Input: part model. Units: mm. Frame: model coordinates. Face numbers are marked on the shaded views. Round coordinates to 2 decimals unless told otherwise and drop trailing zeros. Write each loop counter-clockwise with the first axis right and the second up, starting at its lowest first coordinate (ties: lowest second). Pieces come first, ordered by that corner, then holes. Notation, with made-up numbers: (4.25, 35) - (24.25, 35) arc R29 ccw to (24.25, 65) - close; hole circle Ø10 at (16, 11). An arc over 180 degrees is marked (long way). One line per item, written item: value. Start each with the question number.
```python
from build123d import *

# Parameters (mm, degrees)
SKETCH1_R           = 100
SKETCH1_R_2         = 72.5
BOSS_EXTRUDE1_DEPTH = 8
SKETCH2_R           = 2.25
CUT_EXTRUDE1_DEPTH  = 8


with BuildPart() as part:
    # Sketch1 → Boss-Extrude1 (new body)
    with BuildSketch(Plane(origin=(0, 0, 0), x_dir=(1, 0, 0), z_dir=(0, 1, 0))):
        Circle(SKETCH1_R)
        Circle(SKETCH1_R_2, mode=Mode.SUBTRACT)
    extrude(amount=BOSS_EXTRUDE1_DEPTH)

    # Sketch2 → Cut-Extrude1 (cut)
    with BuildSketch(Plane(origin=(0, 0, 0), x_dir=(1, 0, 0), z_dir=(0, 1, 0))):
        with Locations((0, 93.125)):
            Circle(SKETCH2_R)
        with Locations((93.125, 0)):
            Circle(SKETCH2_R)
        with Locations((0, -93.125)):
            Circle(SKETCH2_R)
        with Locations((-93.125, 0)):
            Circle(SKETCH2_R)
        with Locations((0, 79.375)):
            Circle(SKETCH2_R)
        with Locations((79.375, 0)):
            Circle(SKETCH2_R)
        with Locations((0, -79.375)):
            Circle(SKETCH2_R)
        with Locations((-79.375, 0)):
            Circle(SKETCH2_R)
    extrude(amount=CUT_EXTRUDE1_DEPTH, mode=Mode.SUBTRACT)


solid = part.part
```
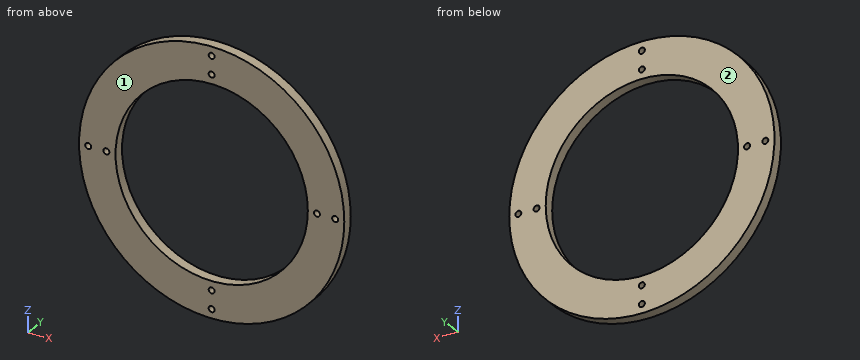
Q1. Cut plane D-D, the plane x = -85. Output: boundary loops of the cut face in (y, z).
Q2. Cut plane B-B, the plane z = 70. Output: boundary loops of the cut face in (x, y), and give its area (3 significant figures).
Q3. Pull-direction query (Y, two-part tool) for the marked faces 1 and 2; classes: pulls with the +Y half, pulls with the -Y half, needs draft (parallel to the pull), parting line crosses it, or undercut.
Q4. Contact query for flat-ended pins moving along their axis: pin 1 Ø2 at (y, z) = (7, 41.5) entering from +X; pin 2 Ø1.5 at (y, z) = (3.5, 32) entering from -X; pin 3 Ø1.5 at (y, z) = (5.5, 55) entering from +X. Output: stop coordinate, or through.
Q5. Cut plane A-A, the plane x = -53. Output: boundary loops of the cut face in (y, z), and give its area (3 significant figures).
Q6. Cut plane C-C, the plane y = 3.75. Count the separate pieces of the cut face and the enclosed holes in it, and give its area (3 significant figures).
Q7. Material intervals for probe 1 along X at (y, z) = (5.75, 0) (3 decimals); probe 2 along Z at (x, y) = (2.5, 6), sorted ascending. Write a range as from..to.
A:
1. outline: (0, -52.68) - (8, -52.68) - (8, 52.68) - (0, 52.68) - close
2. outline: (-71.41, 0) - (-18.87, 0) - (-18.87, 8) - (-71.41, 8) - close; (18.87, 0) - (71.41, 0) - (71.41, 8) - (18.87, 8) - close
2. area: 841 mm²
3. face 1: pulls with the -Y half
3. face 2: pulls with the +Y half
4. pin 1: stops at x = 91.43
4. pin 2: stops at x = -94.99
4. pin 3: stops at x = 84.01
5. outline: (0, -84.8) - (8, -84.8) - (8, -49.47) - (0, -49.47) - close; (0, 49.47) - (8, 49.47) - (8, 84.8) - (0, 84.8) - close
5. area: 565 mm²
6. separate pieces: 1
6. enclosed holes: 9
6. area: 14,800 mm²
7. probe 1: x = -100..-95.375, -90.875..-81.625, -77.125..-72.5, 72.5..77.125, 81.625..90.875, 95.375..100
7. probe 2: z = -99.97..-72.46, 72.46..99.97
